Part model, mm, in its own coordinate system. A direction names the side the tool comes from. Round coordinates to 2 decimals unless told otherwise and drop trailing zeros. Write each loop counter-clockwise with the first axis right and the second up, starting at its lowest first coordinate (ties: lowest second). Pieces come first, ordered by that corner, then holes. Notation, with made-up numbers: M -12.75,-30 L -7.75,-30 A26 ccw -7.75,7 Z; hole C 40,48.25 d11. An arc over 180 degrees is marked long. Use one line per item in the form item = value. Start each with the question number.
Item 1: Which spindle directions (+Z, -Z, +X, -X, +Y, -Y) get a long thin tool onto all of the face, cutting with end or side? Do faces 5 (the face through (45.25, 69, 3)), 6 (the face through (27, 75, 6)), 7 (the face through (47.61, 36.71, 5.86)), 8 (the face through (3.9, 16, 9)). Say none if no direction does.
Item 2: Cut at C-C, the plane y = 10. Give the cut face in (x, z), then the cut area to 3 significant figures.
Item 3: Cut at B-B, the plane x = 27. Give the cut face in (y, z), then the cut area to 4 significant figures.
Item 4: Mould opens along X. For faces 1 (the face through (1, 2, 6)), 2 (the face through (50.3, 16.1, 9.4)), 3 (the face through (27, 0, 6)), 4 (the face through (50.38, 69.19, 5.86)) say: +X half, -X half, draft (parallel to the pull), parting line (faces both ways), or undercut.
Item 5: Cut at A-A, the plane y = 35. Give the cut face in (x, z).
Item 6: Flat gauge pins, fed straight in: pin 1 Ø0.6 at (x, z) = (49.5, 3.5) entering from -Y; pin 2 Ø5 at (x, y) = (39.5, 63) entering from +Z. Where does each tip first touch, or does it go through?
Item 7: Cut at D-D, the plane x = 17. Give the cut face in (y, z), then the cut area to 3 significant figures.
Item 8: Probe L1, parallel to Y at x = 27, z = -0.8; L2, parallel to X at y = 21, z = 12.75; L3, parallel to Y at x = 16.5, z = 3. List the from-to ranges inside material, lowest first.
from build123d import *

# Parameters (mm, degrees)
SKETCH1_W           = 54
SKETCH1_H           = 75
SKETCH1_W_2         = 38
SKETCH1_H_2         = 64
BOSS_EXTRUDE1_DEPTH = 27
CUT_EXTRUDE1_DEPTH  = 4.1
SKETCH5_R           = 4.1
CUT_EXTRUDE2_DEPTH  = 0.5
CUT_EXTRUDE3_DEPTH  = 4.1
SKETCH7_R           = 4.1
CUT_EXTRUDE4_DEPTH  = 0.5
SKETCH8_W           = 54
SKETCH8_H           = 75
BOSS_EXTRUDE2_DEPTH = 2
SKETCH9_W           = 54
SKETCH9_H           = 75
BOSS_EXTRUDE3_DEPTH = 2
SKETCH10_W          = 54
SKETCH10_H          = 75
CUT_EXTRUDE5_DEPTH  = 15.5
SKETCH11_R          = 17.5
CUT_EXTRUDE6_DEPTH  = 3
CUT_EXTRUDE7_DEPTH  = 16.5
SKETCH14_W          = 38
SKETCH14_H          = 5
BOSS_EXTRUDE4_DEPTH = 4
CUT_EXTRUDE8_REACH  = 77
FILLET1_R           = 5


with BuildPart() as part:
    # Sketch1 → Boss-Extrude1 (new body)
    with BuildSketch(Plane.XY):
        with Locations((27, 37.5)):
            Rectangle(SKETCH1_W, SKETCH1_H)
        with Locations((27, 35)):
            Rectangle(SKETCH1_W_2, SKETCH1_H_2, mode=Mode.SUBTRACT)
    extrude(amount=BOSS_EXTRUDE1_DEPTH)

    # Sketch2 → Cut-Extrude1 (cut)
    with BuildSketch(Plane.ZY.offset(-46)):
        Polygon((19.388972746, 54), (16.444486373, 59.1), (10.555513627, 59.1), (7.611027254, 54), (10.555513627, 48.9), (16.444486373, 48.9), align=None)
        Polygon((19.388972746, 16), (16.444486373, 21.1), (10.555513627, 21.1), (7.611027254, 16), (10.555513627, 10.9), (16.444486373, 10.9), align=None)
    extrude(amount=-CUT_EXTRUDE1_DEPTH, mode=Mode.SUBTRACT)

    # Sketch5 → Cut-Extrude2 (cut)
    with BuildSketch(Plane.ZY.offset(-50.1)):
        with Locations((13.5, 54)):
            Circle(SKETCH5_R)
        with Locations((13.5, 16)):
            Circle(SKETCH5_R)
    extrude(amount=-CUT_EXTRUDE2_DEPTH, mode=Mode.SUBTRACT)

    # Sketch6 → Cut-Extrude3 (cut)
    with BuildSketch(Plane(origin=(8, 0, 0), x_dir=(0, 0, -1), z_dir=(1, 0, 0))):
        Polygon((-7.611027254, 54), (-10.555513627, 59.1), (-16.444486373, 59.1), (-19.388972746, 54), (-16.444486373, 48.9), (-10.555513627, 48.9), align=None)
        Polygon((-7.611027254, 16), (-10.555513627, 21.1), (-16.444486373, 21.1), (-19.388972746, 16), (-16.444486373, 10.9), (-10.555513627, 10.9), align=None)
    extrude(amount=-CUT_EXTRUDE3_DEPTH, mode=Mode.SUBTRACT)

    # Sketch7 → Cut-Extrude4 (cut)
    with BuildSketch(Plane(origin=(3.9, 0, 0), x_dir=(0, 0, -1), z_dir=(1, 0, 0))):
        with Locations((-13.5, 54)):
            Circle(SKETCH7_R)
        with Locations((-13.5, 16)):
            Circle(SKETCH7_R)
    extrude(amount=-CUT_EXTRUDE4_DEPTH, mode=Mode.SUBTRACT)

    # Sketch8 → Boss-Extrude2 (add)
    with BuildSketch(Plane.XY.offset(27)):
        with Locations((27, 37.5)):
            Rectangle(SKETCH8_W, SKETCH8_H)
    extrude(amount=BOSS_EXTRUDE2_DEPTH)

    # Sketch9 → Boss-Extrude3 (add)
    with BuildSketch(Plane(origin=(0, 0, 0), x_dir=(-1, 0, 0), z_dir=(0, 0, -1))):
        with Locations((-27, 37.5)):
            Rectangle(SKETCH9_W, SKETCH9_H)
    extrude(amount=BOSS_EXTRUDE3_DEPTH)

    # Sketch10 → Cut-Extrude5 (cut)
    with BuildSketch(Plane.XY.offset(29)):
        with Locations((27, 37.5)):
            Rectangle(SKETCH10_W, SKETCH10_H)
    extrude(amount=-CUT_EXTRUDE5_DEPTH, mode=Mode.SUBTRACT)

    # Sketch11 → Cut-Extrude6 (cut, through all)
    with BuildSketch(Plane.XY):
        with Locations((27, 35)):
            Circle(SKETCH11_R)
    extrude(amount=-CUT_EXTRUDE6_DEPTH, mode=Mode.SUBTRACT)

    # Sketch12 → Cut-Extrude7 (cut, through all)
    with BuildSketch(Plane.XY.offset(13.5)):
        Polygon((6.443375673, 70), (5.721687836, 71.25), (4.278312164, 71.25), (3.556624327, 70), (4.278312164, 68.75), (5.721687836, 68.75), align=None)
        Polygon((50.847520861, 70), (49.923760431, 71.6), (48.076239569, 71.6), (47.152479139, 70), (48.076239569, 68.4), (49.923760431, 68.4), align=None)
        Polygon((6.443375673, 5), (5.721687836, 6.25), (4.278312164, 6.25), (3.556624327, 5), (4.278312164, 3.75), (5.721687836, 3.75), align=None)
        Polygon((50.847520861, 5), (49.923760431, 6.6), (48.076239569, 6.6), (47.152479139, 5), (48.076239569, 3.4), (49.923760431, 3.4), align=None)
        Polygon((50.847520861, 37.5), (49.923760431, 39.1), (48.076239569, 39.1), (47.152479139, 37.5), (48.076239569, 35.9), (49.923760431, 35.9), align=None)
        Polygon((6.443375673, 37.5), (5.721687836, 38.75), (4.278312164, 38.75), (3.556624327, 37.5), (4.278312164, 36.25), (5.721687836, 36.25), align=None)
    extrude(amount=-CUT_EXTRUDE7_DEPTH, mode=Mode.SUBTRACT)

    # Sketch14 → Boss-Extrude4 (add)
    with BuildSketch(Plane.XZ.offset(-67)):
        with Locations((27, 2.5)):
            Rectangle(SKETCH14_W, SKETCH14_H)
    extrude(amount=BOSS_EXTRUDE4_DEPTH)

    # Sketch13 → Cut-Extrude8 (cut, up to next)
    with BuildSketch(Plane(origin=(0, 75, 0), x_dir=(1, 0, 0), z_dir=(0, 1, 0)), mode=Mode.PRIVATE) as cut_extrude8_sk1:
        Polygon((44, -1.056624327), (42.75, -1.778312164), (42.75, -3.221687836), (44, -3.943375673), (45.25, -3.221687836), (45.25, -1.778312164), align=None)
    cut_extrude8_tool1 = extrude(cut_extrude8_sk1.sketch, amount=-CUT_EXTRUDE8_REACH, mode=Mode.PRIVATE) & part.part
    add(cut_extrude8_tool1.solids().sort_by_distance((44, 75, 2.5))[0], mode=Mode.SUBTRACT)
    # Sketch13 → Cut-Extrude8 (cut, up to next)
    with BuildSketch(Plane(origin=(0, 75, 0), x_dir=(1, 0, 0), z_dir=(0, 1, 0)), mode=Mode.PRIVATE) as cut_extrude8_sk2:
        Polygon((10, -1.056624327), (8.75, -1.778312164), (8.75, -3.221687836), (10, -3.943375673), (11.25, -3.221687836), (11.25, -1.778312164), align=None)
    cut_extrude8_tool2 = extrude(cut_extrude8_sk2.sketch, amount=-CUT_EXTRUDE8_REACH, mode=Mode.PRIVATE) & part.part
    add(cut_extrude8_tool2.solids().sort_by_distance((10, 75, 2.5))[0], mode=Mode.SUBTRACT)

    # Fillet1
    fillet1_edges = [part.edges().sort_by_distance(p)[0] for p in [
        (0, 0, 5.75),
        (54, 0, 5.75),
    ]]
    fillet(fillet1_edges, radius=FILLET1_R)


solid = part.part
Model answer:
q1.face_5 = +Y
q1.face_6 = +Z, -Z, +X, -X, +Y
q1.face_7 = +Z, -Z
q1.face_8 = +Z
q2.outline = M 0,-2 L 54,-2 L 54,13.5 L 46,13.5 L 46,0 L 8,0 L 8,13.5 L 0,13.5 Z
q2.area = 324 mm²
q3.outline = M 0,-2 L 17.5,-2 L 17.5,0 L 3,0 L 3,13.5 L 0,13.5 Z; M 52.5,-2 L 75,-2 L 75,13.5 L 67,13.5 L 67,5 L 63,5 L 63,0 L 52.5,0 Z
q3.area = 248.5 mm²
q4.face_1 = -X half
q4.face_2 = undercut
q4.face_3 = draft
q4.face_4 = undercut
q5.outline = M 0,-2 L 9.5,-2 L 9.5,0 L 8,0 L 8,13.5 L 0,13.5 Z; M 44.5,-2 L 54,-2 L 54,13.5 L 46,13.5 L 46,0 L 44.5,0 Z
q6.pin_1 = 0
q6.pin_2 = 5
q7.outline = M 0,-2 L 20.64,-2 L 20.64,0 L 3,0 L 3,13.5 L 0,13.5 Z; M 49.36,-2 L 75,-2 L 75,13.5 L 67,13.5 L 67,5 L 63,5 L 63,0 L 49.36,0 Z
q7.area = 261 mm²
q8.L1 = 0 to 17.5, 52.5 to 75
q8.L2 = 0 to 3.9, 50.1 to 54
q8.L3 = 0 to 3, 63 to 75
